from build123d import *

# Parameters (mm, degrees)
SKETCH1_W           = 465
SKETCH1_H           = 254
BOSS_EXTRUDE1_DEPTH = 2
SKETCH2_W           = 50
SKETCH2_H           = 12
CUT_EXTRUDE1_DEPTH  = 2
SKETCH3_W           = 6
SKETCH3_H           = 60
BOSS_EXTRUDE2_DEPTH = 2
SKETCH4_W           = 50
SKETCH4_H           = 25
CUT_EXTRUDE2_DEPTH  = 2


with BuildPart() as part:
    # Sketch1 → Boss-Extrude1 (new body)
    with BuildSketch(Plane.XY):
        Rectangle(SKETCH1_W, SKETCH1_H)
    extrude(amount=BOSS_EXTRUDE1_DEPTH)

    # Sketch2 → Cut-Extrude1 (cut)
    with BuildSketch(Plane.XY.offset(2)):
        with Locations((-139.5, -127)):
            Rectangle(SKETCH2_W, SKETCH2_H)
        with Locations((-46.5, -127)):
            Rectangle(SKETCH2_W, SKETCH2_H)
        with Locations((46.5, -127)):
            Rectangle(SKETCH2_W, SKETCH2_H)
        with Locations((139.5, -127)):
            Rectangle(SKETCH2_W, SKETCH2_H)
        with Locations((-139.5, 127)):
            Rectangle(SKETCH2_W, SKETCH2_H)
        with Locations((-46.5, 127)):
            Rectangle(SKETCH2_W, SKETCH2_H)
        with Locations((46.5, 127)):
            Rectangle(SKETCH2_W, SKETCH2_H)
        with Locations((139.5, 127)):
            Rectangle(SKETCH2_W, SKETCH2_H)
    extrude(amount=-CUT_EXTRUDE1_DEPTH, mode=Mode.SUBTRACT)

    # Sketch3 → Boss-Extrude2 (add)
    with BuildSketch(Plane.XY.offset(2)):
        with Locations((-235.5, 97)):
            Rectangle(SKETCH3_W, SKETCH3_H)
        with Locations((235.5, 97)):
            Rectangle(SKETCH3_W, SKETCH3_H)
    extrude(amount=-BOSS_EXTRUDE2_DEPTH)

    # Sketch4 → Cut-Extrude2 (cut)
    with BuildSketch(Plane.XY.offset(2)):
        with Locations((-139.5, -108.5)):
            Rectangle(SKETCH4_W, SKETCH4_H)
        with Locations((46.5, -108.5)):
            Rectangle(SKETCH4_W, SKETCH4_H)
        with Locations((139.5, -108.5)):
            Rectangle(SKETCH4_W, SKETCH4_H)
        with Locations((-46.5, -108.5)):
            Rectangle(SKETCH4_W, SKETCH4_H)
    extrude(amount=-CUT_EXTRUDE2_DEPTH, mode=Mode.SUBTRACT)


solid = part.part
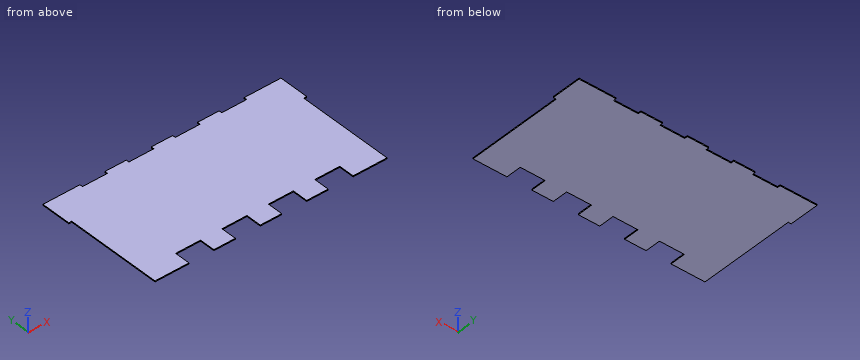
The listing builds one solid part. Answer for the finished solid, in the listing's coordinates (mm). Coordinates: 2 decimals unless noted, no trailing zeros. Write each loop counter-clockwise with the first axis right and the second up, starting at its lowest first coordinate (ties: lowest second). Pieces come first, ordered by that corner, then holes. Notation, with made-up numbers: (50.5, -34.75) -> (73.5, -34.75) arc R22 cw to (73.5, -26.75) -> close; hole circle Ø9 at (-13, -9). An arc over 180 degrees is marked (long way). One line per question, with ' | ' between items.
1. Straight lines are drawn through the part: line 1 (X direction, y = -113.5, z = 0.55); line 2 (X direction, y = -5, z = 1.05); line 3 (Y direction, x = -129, z = 1.45). For each, find the intervals that lie inside material, in ascending order.
Verdict:
line 1: x = -232.5 to -164.5, -114.5 to -71.5, -21.5 to 21.5, 71.5 to 114.5, 164.5 to 232.5 | line 2: x = -232.5 to 232.5 | line 3: y = -96 to 121
2. Given pin 1 Ø1 at (x, z) = (236, 1.5) entering from -Y; pin 2 Ø1 at (x, y) = (82.5, -20.5) entering from -Z; pin 3 Ø0.6 at (x, z) = (-131, 1) entering from -Y; pin 4 Ø1 at (y, z) = (-110.5, 1) entering from +X, each flat-ended and moving along its own axis, determine where each tip first touches the part or whether it passes through.
Verdict:
pin 1: stops at y = 67 | pin 2: stops at z = 0 | pin 3: stops at y = -96 | pin 4: stops at x = 232.5
3. Section A-A (x = -44.5) is taken. Determine the outline of the cut face in (y, z), and give its area (3 significant figures).
Verdict:
outline: (-96, 0) -> (121, 0) -> (121, 2) -> (-96, 2) -> close | area: 434 mm^2
4. Section B-B (y = 39) is taken. Determine the outline of the cut face in (x, z), and give its area (3 significant figures).
Verdict:
outline: (-232.5, 0) -> (232.5, 0) -> (232.5, 2) -> (-232.5, 2) -> close | area: 930 mm^2
